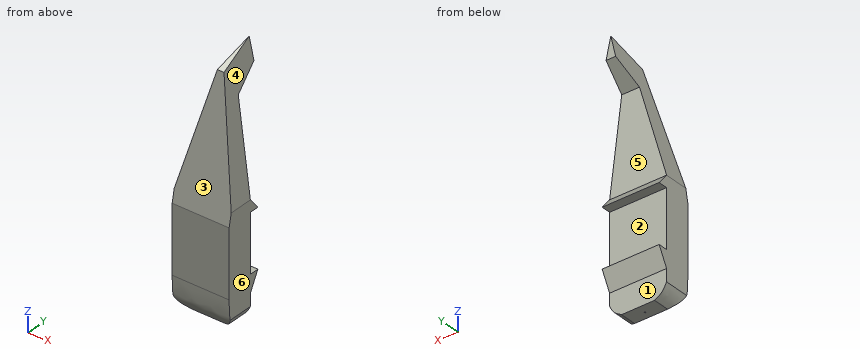
from build123d import *

# Parameters (mm, degrees)
F0_W     = 200
F0_H     = 272
F1_DEPTH = 414
F3_DEPTH = 200.001
F5_DEPTH = 214.0125203069
F7_D     = 5
F7_DEPTH = 50
F7_TIP   = 1.5021515476


with BuildPart() as f1:
    # F0 (on Top) → F1 (new body, symmetric)
    with BuildSketch(Plane.XY):
        Rectangle(F0_W, F0_H)
    extrude(amount=F1_DEPTH, both=True)

    # F2 (on face) → F3 (cut, through all)
    with BuildSketch(Plane(origin=(-100, 0, 0), x_dir=(0, -1, 0), z_dir=(-1, 0, 0))):
        Polygon((-48.6409515142, 278.2896161079), (-136, 340.7483696938), (-136, -414), (-15.6766073778, -414), (-15.6766073778, -326.6927754041), (-48.640947789, -264.7544890642), (-15.6766073778, -264.7544890642), (-15.6766073778, -61.7635734379), (-48.640947789, -61.7635734379), (-15.6766073778, -21.04292392), align=None)
        with BuildLine():
            Line((136, 414), (-136, 414))
            Line((-136, 414), (-10.4717324721, 363.3029013872))
            Line((-10.4717324721, 363.3029013872), (78.0115202069, -65.2334988117))
            Line((78.0115202069, -65.2334988117), (78.0115202069, -301.1887669563))
            add(Edge.make_bspline(
                [(41.577257216, -414), (52.5528446959, -402.42919259), (72.8831837624, -381.0445803549), (76.791037733, -347.6423075278), (78.0115202069, -317.6310269751), (78.0115202069, -301.1887669563)],
                knots=[0, 0, 0, 0, 0.3478343827, 0.6428666129, 1, 1, 1, 1], degree=3))
            Line((41.577257216, -414), (136, -414))
            Line((136, -414), (136, 414))
        make_face()
    extrude(amount=-F3_DEPTH, mode=Mode.SUBTRACT)

    # F4 (on face) → F5 (cut, through all)
    with BuildSketch(Plane.XZ.offset(78.0115202069)):
        Polygon((-100, -21.04292392), (0, 414), (-100, 414), (-100, 340.7483696938), (-100, 278.2896161079), align=None)
        Polygon((100, 414), (0, 414), (100, -21.04292392), (100, 278.2896161079), (100, 340.7483696938), align=None)
        with BuildLine():
            Line((57.925209403, -414), (100, -414))
            Line((100, -414), (100, -370.346387702))
            add(Edge.make_bspline(
                [(100, -370.346387702), (95.4592593145, -379.6018433489), (86.2772620908, -398.3176375197), (67.4446143257, -408.7345343832), (57.925209403, -414)],
                knots=[0, 0, 0, 0, 0.4945264712, 1, 1, 1, 1], degree=3))
        make_face()
        with BuildLine():
            Line((-100, -414), (-57.925209403, -414))
            add(Edge.make_bspline(
                [(-100, -370.346387702), (-95.4592593145, -379.6018433489), (-86.2772620908, -398.3176375197), (-67.4446143257, -408.7345343832), (-57.925209403, -414)],
                knots=[0, 0, 0, 0, 0.4945264712, 1, 1, 1, 1], degree=3))
            Line((-100, -370.346387702), (-100, -414))
        make_face()
    extrude(amount=-F5_DEPTH, mode=Mode.SUBTRACT)

    # F7
    with Locations(Plane(origin=(0, 0, -414), x_dir=(1, 0, 0), z_dir=(0, 0, -1))):
        with Locations((0, 15.3372772038)):
            Hole(F7_D / 2, depth=F7_DEPTH)
            with Locations((0, 0, -(F7_DEPTH + F7_TIP / 2))):  # 118° drill point
                Cone(0, F7_D / 2, F7_TIP, mode=Mode.SUBTRACT)


solid = f1.part
Check sheet for the modelled part. Datum: model origin and axes. Units: mm. Face numbers are marked on the shaded views. A direction names the side the tool comes from. Round coordinates to 2 decimals unless told otherwise and drop trailing zeros. Order: outer loops, then holes, each group sorted by start corner. A loop starts at its lowest first (then second) coordinate and runs counter-clockwise, first axis right, second up. Notation, with made-up numbers: M -38.75,-10.75 L 3.25,-10.75 A19 cw 3.25,26.25 Z; hole C -22,4.5 d8. An arc over 180 degrees is marked long. One line per item, written item: value. Start each with the question number.
1. Section check B-B on y = 117. Enter the section's corners in (x, z).
2. Scan lines: line 1 along Y through (x, z) = (-63, -225.5); line 2 along Y through (x, z) = (0, -394); line 3 along Y through (x, z) = (0, -387). Record each from-to range of solid material in increasing order.
3. Section check A-A on z = -280. Enter the section's corners in (x, y), and give its area (3 significant figures).
4. Release check for a two-part mould opening along Z. For the marked faces 4, 5 and 6 record: released by +Z, released by -Z, zero draft, split by the parting line, or undercut.
5. Access from +Z, -Z, +X, -X, +Y, -Y to the whole of each face (thin tool, end or side, straight path). Record for the marked faces 1, 2 and 3.
6. Gauge pin test, flat ends, axial feed: P1, Ø12, axis at y = -3.5, z = 91, coming from the +X side; P2, Ø5, axis at x = 43, z = 145.5, coming from the +Y side; P3, Ø2, axis at x = 51.5, y = 50.5, coming from the -Z side; P4, Ø10, axis at x = -40.5, y = 31, coming from the -Z side. Record the tip position at first contact, or that the pin passes through.
Results found:
1. outline: M -19.96,327.16 L 19.96,327.16 L 1.76,406.33 L -1.76,406.33 Z
2. line 1: -78.01 to 15.68
2. line 2: -59.57 to -17.84, -12.84 to 15.68
2. line 3: -64.76 to -17.84, -12.84 to 15.68
3. outline: M -100,-78.01 L 100,-78.01 L 100,40.53 L -100,40.53 Z
3. area: 23,700 mm^2
4. face 4: released by +Z
4. face 5: undercut
4. face 6: zero draft
5. face 1: -Z, +X, -X, +Y
5. face 2: +X, -X, +Y
5. face 3: +Z, +X, -X, -Y
6. P1: x = 75.62
6. P2: y = 34.29
6. P3: through
6. P4: z = -307.3
